```python
from build123d import *

# Parameters (mm, degrees)
SKETCH1_W            = 26.4
SKETCH1_H            = 26.4
BOSS_EXTRUDE1_DEPTH  = 117
SKETCH60_W           = 48
SKETCH60_H           = 40
CUT_EXTRUDE1_DEPTH   = 87
CUT_EXTRUDE2_DEPTH   = 157.009486891
M4_CLEARANCE_HOLE1_D = 4.8
SKETCH66_W           = 48
SKETCH66_H           = 31.290838495
CUT_EXTRUDE3_DEPTH   = 40
CUT_EXTRUDE5_DEPTH   = 157.009486891
SKETCH69_W           = 98
SKETCH69_H           = 56
CUT_EXTRUDE6_DEPTH   = 144.174578749
SKETCH70_W           = 6
SKETCH70_H           = 7
CUT_EXTRUDE7_DEPTH   = 136.066502139


with BuildPart() as part:
    # Sketch1 → Boss-Extrude1 (new body)
    with BuildSketch(Plane.XY):
        Polygon((-3, -41.4), (3, -41.4), (16, -54.4), (24, -54.4), (24, -66.4), (49, -66.4), (49, -61.4), (30, -61.4), (30, 5), (-30, 5), (-30, -61.4), (-49, -61.4), (-49, -66.4), (-24, -66.4), (-24, -54.4), (-16, -54.4), align=None)
        with Locations((0, -13.2)):
            Rectangle(SKETCH1_W, SKETCH1_H, mode=Mode.SUBTRACT)
    extrude(amount=BOSS_EXTRUDE1_DEPTH)

    # Sketch60 → Cut-Extrude1 (cut)
    with BuildSketch(Plane(origin=(0, 0, 0), x_dir=(-1, 0, 0), z_dir=(0, 0, -1))):
        with Locations((0, -15)):
            Rectangle(SKETCH60_W, SKETCH60_H)
    extrude(amount=-CUT_EXTRUDE1_DEPTH, mode=Mode.SUBTRACT)

    # Sketch61 → Cut-Extrude2 (cut, through all)
    with BuildSketch(Plane.ZY.offset(30)):
        Polygon((0, -43.4), (38, -43.4), (56, -61.4), (0, -61.4), align=None)
    extrude(amount=-CUT_EXTRUDE2_DEPTH, mode=Mode.SUBTRACT)

    # M4 Clearance Hole1 (through all)
    with Locations(Plane.ZY.offset(30)):
        with Locations((5.25, -14.37), (5.25, -26.77), (21.8, -34.86)):
            Hole(M4_CLEARANCE_HOLE1_D / 2)

    # Sketch66 → Cut-Extrude3 (cut)
    with BuildSketch(Plane(origin=(0, 0, 0), x_dir=(-1, 0, 0), z_dir=(0, 0, -1))):
        with Locations((0, -50.645419248)):
            Rectangle(SKETCH66_W, SKETCH66_H)
    extrude(amount=-CUT_EXTRUDE3_DEPTH, mode=Mode.SUBTRACT)

    # Sketch68 → Cut-Extrude5 (cut, through all)
    with BuildSketch(Plane.ZY.offset(30)):
        Polygon((22.733334145, -0.733334145), (57, -35), (87, -35), (87, 5), (22.733334145, 5), align=None)
    extrude(amount=-CUT_EXTRUDE5_DEPTH, mode=Mode.SUBTRACT)

    # Sketch69 → Cut-Extrude6 (cut, through all)
    with BuildSketch(Plane(origin=(0, -61.4, 0), x_dir=(1, 0, 0), z_dir=(0, 1, 0))):
        with Locations((0, -28)):
            Rectangle(SKETCH69_W, SKETCH69_H)
    extrude(amount=-CUT_EXTRUDE6_DEPTH, mode=Mode.SUBTRACT)

    # Sketch70 → Cut-Extrude7 (cut, through all)
    with BuildSketch(Plane.XZ.offset(41.4)):
        with Locations((0, 43.5)):
            Rectangle(SKETCH70_W, SKETCH70_H)
    extrude(amount=-CUT_EXTRUDE7_DEPTH, mode=Mode.SUBTRACT)


solid = part.part
```
Verification items for the finished model (mm, model axes). A direction names the side the tool comes from. Coordinates: 2 decimals unless noted, no trailing zeros. Order: outer loops, then holes, each group sorted by start corner. A loop starts at its lowest first (then second) coordinate and runs counter-clockwise, first axis right, second up. Notation, with made-up numbers: (58.25, 64) - (106.25, 64) arc R7 cw to (106.25, 71) - close; hole circle Ø1 at (-11, 63). An arc over 180 degrees is marked (long way). Return JSON: item names as keys, results as strings.
(1) Section check D-D, the plane x = -22. Record the cut outline in (y, z).
Filled sheet:
{"outline": "(-54.4, 49) - (-45.4, 40) - (-35, 40) - (-35, 87) - (5, 87) - (5, 117) - (-54.4, 117) - close"}
(2) Section check A-A, the plane z = 5.25. Record the cut outline in (x, y), and give its area (3 significant figures).
Filled sheet:
{"outline": "(-30, -43.4) - (-24, -43.4) - (-24, -29.17) - (-30, -29.17) - close; (-30, -24.37) - (-24, -24.37) - (-24, -16.77) - (-30, -16.77) - close; (-30, -11.97) - (-24, -11.97) - (-24, 5) - (-30, 5) - close; (24, -43.4) - (30, -43.4) - (30, -29.17) - (24, -29.17) - close; (24, -24.37) - (30, -24.37) - (30, -16.77) - (24, -16.77) - close; (24, -11.97) - (30, -11.97) - (30, 5) - (24, 5) - close", "area": "466 mm^2"}
(3) Thickness scan on line 1 along Y through (x, z) = (26.35, 5.25); line 2 along Z through (x, y) = (-28.5, -27); line 3 along X through (y, z) = (-4.5, 106). Record the ranges inside material, lowest first.
Filled sheet:
{"line 1": "y = -43.4 to -29.17, -24.37 to -16.77, -11.97 to 5", "line 2": "z = 0 to 2.86, 7.64 to 49, 87 to 117", "line 3": "x = -30 to -13.2, 13.2 to 30"}
(4) Access from +Z, -Z, +X, -X, +Y, -Y to the whole of each face (thin tool, end or side, straight path). Record for faces 5 (the flat face through (-3, -38, 43)), 6 (the flat face through (0, -41.4, 82)), 7 (the flat face through (27, -43.4, 19)), 8 (the flat face through (-39, -61.4, 86)), 9 (the flat face through (-27, -18, 40)).
Filled sheet:
{"face 5": "-Z, +Y, -Y", "face 6": "+Z, -Z, -Y", "face 7": "-Z, +X, -X, -Y", "face 8": "+Z, -Z, -X, +Y", "face 9": "+X, -X, +Y"}
(5) Section check C-C, the plane z = 17.5. Record the cut outline in (x, y).
Filled sheet:
{"outline": "(-30, -43.4) - (-24, -43.4) - (-24, 5) - (-30, 5) - close; (24, -43.4) - (30, -43.4) - (30, 5) - (24, 5) - close"}
(6) Section check B-B, the plane y = -8.5. Record the cut outline in (x, z), and give its area (3 significant figures).
Filled sheet:
{"outline": "(-30, 0) - (-24, 0) - (-24, 30.5) - (-30, 30.5) - close; (-30, 87) - (-13.2, 87) - (-13.2, 117) - (-30, 117) - close; (13.2, 87) - (30, 87) - (30, 117) - (13.2, 117) - close; (24, 0) - (30, 0) - (30, 30.5) - (24, 30.5) - close", "area": "1,370 mm^2"}
(7) Go/stop test with flat-tipped pins: pin 1 (2 mm diameter, centred on x = 1.5, y = -29, fed in from -Z); pin 2 (21 mm diameter, centred on x = -6.5, z = 107.5, fed in from -Y); pin 3 (5.5 mm diameter, centred on y = -26.77, z = 5.25, fed in from -X). Record where each tip stops, or that it passes through.
Filled sheet:
{"pin 1": "stops at z = 87", "pin 2": "stops at y = -54.4", "pin 3": "stops at x = -30"}
(8) Mould release check, pull along X, two halves, no side actions. Record for faces 1 (the flat face through (27, 2, 22.733)), 2 (the flat face through (-13.2, -13, 102)), 3 (the flat face through (49, -64, 86)), 4 (the flat face through (-49, -64, 86)): pulls with the +X half, pulls with the -X half, needs draft (parallel to the pull), parting line crosses it, or undercut.
Filled sheet:
{"face 1": "needs draft", "face 2": "undercut", "face 3": "pulls with the +X half", "face 4": "pulls with the -X half"}
